```python
from build123d import *

# Parameters (mm, degrees)
F0_W     = 10
F0_H     = 20
F1_DEPTH = 16
F2_D     = 8
F4_D     = 4
F5_R     = 3


with BuildPart() as f1:
    # F0 (on Front) → F1 (new body)
    with BuildSketch(Plane.XZ):
        with BuildLine():
            Line((-8, 2.5), (-22, 2.5))
            Line((-22, 2.5), (-22, -2.5))
            Line((-22, -2.5), (22, -2.5))
            Line((22, -2.5), (22, 2.5))
            Line((22, 2.5), (8, 2.5))
            Line((8, 2.5), (8, 36.5))
            ThreePointArc((8, 36.5), (0, 44.5), (-8, 36.5))
            Line((-8, 36.5), (-8, 2.5))
        make_face()
        with Locations((0, 16.5)):
            Rectangle(F0_W, F0_H, mode=Mode.SUBTRACT)
    extrude(amount=F1_DEPTH)

    # F2 (through all)
    with Locations(Plane(origin=(0, 0, 0), x_dir=(1, 0, 0), z_dir=(0, 1, 0))):
        with Locations((0, -36.5)):
            Hole(F2_D / 2)

    # F4 (through all)
    with Locations(Plane(origin=(0, 0, -2.5), x_dir=(1, 0, 0), z_dir=(0, 0, -1))):
        with Locations((-16, 8), (16, 8)):
            Hole(F4_D / 2)

    # F5
    f5_edges = [f1.edges().sort_by_distance(p)[0] for p in [
        (-8, -8, 2.5),
        (8, -8, 2.5),
        (5, -8, 6.5),
        (-5, -8, 6.5),
        (-5, -8, 26.5),
        (5, -8, 26.5),
    ]]
    fillet(f5_edges, radius=F5_R)


solid = f1.part
```
The listing builds one solid part. Answer for the finished solid, in the listing's coordinates (mm). A direction names the side the tool comes from. Coordinates: 2 decimals unless noted, no trailing zeros. Write each loop counter-clockwise with the first axis right and the second up, starting at its lowest first coordinate (ties: lowest second). Pieces come first, ordered by that corner, then holes. Notation, with made-up numbers: (-25, -38.5) - (-14, -38.5) arc R25 cw to (-14, -4.5) - close; hole circle Ø7 at (13, 28.25). An arc over 180 degrees is marked (long way). Return JSON: item names as keys, results as strings. Group by question number.
Q1. Find the intervals of material crossed by line 1 along X through (y, z) = (-11.75, 16); line 2 along Y through (x, z) = (16, -1.3); line 3 along Z through (x, y) = (0, -6.25), in increasing order. Write a range as [from, to].
Q2. Which of the six approach directions +Z, -Z, +X, -X, +Y, -Y give full straight-line access (tool end or side, diameter ignored) to faces 4 (the flat face through (-18, -6, 2.5)), 5 (the flat face through (0, -8, -2.5)), 6 (the flat face through (8, -8, 21)), 7 (the cylindrical face through (17.474, -9.352, 0.035)), 8 (the flat face through (5, -8, 16))?
Q3. The part is cut by section A-A on z = 15.5. Write down the section's boundary in (x, y).
Q4. Flat-ended cylindrical pins translate along their axes: pin 1 Ø1 at (y, z) = (-6, 18) entering from +X; pin 2 Ø9 at (x, y) = (17, -11) entering from +Z; pin 3 Ø1 at (y, z) = (-6.5, 15) entering from -X; pin 4 Ø3.5 at (x, y) = (-16, -8) entering from +Z. Find the tip coordinate at first contact, or state that the pin passes through.
Q5. The part is cut by section B-B on y = -8. Write down the section's boundary in (x, z).
Q6. The part is cut by section D-D on y = -1.5. Write down the section's boundary in (x, z), and give its area (3 significant figures).
Q7. The part is cut by section C-C on x = 16. Write down the section's boundary in (y, z), and give its area (3 significant figures).
Q8. For a pull along Z with two mould halves and no side action, classify faces 1 (the flat face through (0, -8, 6.5)), 2 (the flat face through (-8, -8, 21)), 3 (the cylindrical face through (-8.9, -8.11, 3.36)) as +Z half, -Z half, draft (parallel to the pull), parting line (faces both ways), or undercut.
Evaluation:
{
 "1": {"line 1": "x = [-8, -5], [5, 8]", "line 2": "y = [-16, -10], [-6, 0]", "line 3": "z = [-2.5, 6.5], [26.5, 32.5], [40.5, 44.5]"},
 "2": {"face 4": "+Z, -X, +Y, -Y", "face 5": "-Z, +X, -X, +Y, -Y", "face 6": "+Z, +X, +Y, -Y", "face 7": "+Z, -Z", "face 8": "+Y, -Y"},
 "3": {"outline": "(-8, -16) - (-5, -16) - (-5, 0) - (-8, 0) - close; (5, -16) - (8, -16) - (8, 0) - (5, 0) - close"},
 "4": {"pin 1": "stops at x = 8", "pin 2": "stops at z = 2.5", "pin 3": "stops at x = -8", "pin 4": "passes through"},
 "5": {"outline": "(-22, -2.5) - (-18, -2.5) - (-18, 2.5) - (-22, 2.5) - close; (-14, -2.5) - (14, -2.5) - (14, 2.5) - (11, 2.5) arc R3 cw to (8, 5.5) - (8, 36.5) arc R8 ccw to (-8, 36.5) - (-8, 5.5) arc R3 cw to (-11, 2.5) - (-14, 2.5) - close; (18, -2.5) - (22, -2.5) - (22, 2.5) - (18, 2.5) - close; hole (-5, 9.5) arc R3 ccw to (-2, 6.5) - (2, 6.5) arc R3 ccw to (5, 9.5) - (5, 23.5) arc R3 ccw to (2, 26.5) - (-2, 26.5) arc R3 ccw to (-5, 23.5) - close; hole circle Ø8 at (0, 36.5)"},
 "6": {"outline": "(-22, -2.5) - (22, -2.5) - (22, 2.5) - (11, 2.5) arc R3 cw to (8, 5.5) - (8, 36.5) arc R8 ccw to (-8, 36.5) - (-8, 5.5) arc R3 cw to (-11, 2.5) - (-22, 2.5) - close; hole (-5, 9.5) arc R3 ccw to (-2, 6.5) - (2, 6.5) arc R3 ccw to (5, 9.5) - (5, 23.5) arc R3 ccw to (2, 26.5) - (-2, 26.5) arc R3 ccw to (-5, 23.5) - close; hole circle Ø8 at (0, 36.5)", "area": "626 mm2"},
 "7": {"outline": "(-16, -2.5) - (-10, -2.5) - (-10, 2.5) - (-16, 2.5) - close; (-6, -2.5) - (0, -2.5) - (0, 2.5) - (-6, 2.5) - close", "area": "60.0 mm2"},
 "8": {"face 1": "undercut", "face 2": "draft", "face 3": "+Z half"}
}
